Geometry: final body of the model. Coordinates: model frame, mm. Face numbers are marked on the shaded views. A direction names the side the tool comes from. Give positions to 0.01 mm unless a question says otherwise; leave off trailing zeros. Loops run counter-clockwise (first coordinate to the right, second up) from the corner with the lowest first, then second, coordinate; pieces in that order, holes last.
1. Section B-B, the plane y = 0. Output: boundary loops of the cut face in (x, z).
2. Access query for the marked faces 5, 6 and 7. Directions: +Z, -Z, +X, -X, +Y, -Y. A direction counts if a zero-diameter tool reaches every point of the face in a straight line with its end or side. Return the directions, or none.
3. Material intervals for line 1 along Z through (x, y) = (-16, -11); line 2 along Z through (x, y) = (-53, 55); line 3 along X through (y, z) = (60, -5.5), sorted ascending.
4. Draft query along Z for the marked faces 1, 2, 3 and 4. Return one class per face: +Z half, -Z half, draft (parallel to the pull), parting line (faces both ways), or undercut.
5. Section A-A, the plane x = -10. Output: boundary loops of the cut face in (y, z), then the cut area to 3 significant figures.
6. Section D-D, the plane x = -62.5. Output: boundary loops of the cut face in (y, z).
7. Section C-C, the plane z = -20. Output: boundary loops of the cut face in (x, y), then the cut area to 3 significant figures.
8. First-contact query: P1, Ø22, axis at x = -27.5, y = 18, coming from the +Z side; P2, Ø6, axis at x = -55.5, y = 23, coming from the +Z side; P3, Ø1, axis at x = -36.5, y = 46.5, coming from the -Z side; P4, Ø1, axis at y = 38.5, z = -32.5, coming from the +X side. Flat tips, straight axial feed; report the tip coordinate or a pass-through.
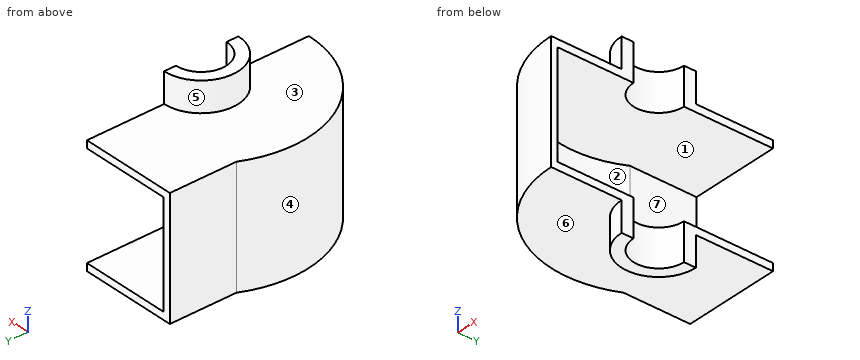
from build123d import *

# Parameters (mm, degrees)
BOSS_EXTRUDE1_DEPTH      = 20
BOSS_EXTRUDE1_DEPTH_BACK = 5
BOSS_EXTRUDE3_DEPTH      = 5
BOSS_EXTRUDE4_DEPTH      = 75


with BuildPart() as part:
    # Sketch1 → Boss-Extrude1 (new body, two sides)
    with BuildSketch(Plane.XY) as boss_extrude1_sk:
        with BuildLine():
            Line((0, 25), (0, 17))
            ThreePointArc((0, 17), (-17, 0), (0, -17))
            Line((0, -17), (0, -25))
            ThreePointArc((0, -25), (-25, 0), (0, 25))
        make_face()
    extrude(amount=BOSS_EXTRUDE1_DEPTH)
    extrude(boss_extrude1_sk.sketch, amount=-BOSS_EXTRUDE1_DEPTH_BACK)

    # Sketch2 → Boss-Extrude3 (add)
    with BuildSketch(Plane.XY):
        with BuildLine():
            Line((0, 25), (0, 77))
            Line((0, 77), (-65, 77))
            Line((-65, 77), (-65, 32.113081447))
            ThreePointArc((-65, 32.113081447), (-61.581037686, -38.262590053), (0, -72.5))
            Line((0, -72.5), (0, -25))
            ThreePointArc((0, -25), (-25, 0), (0, 25))
        make_face()
    extrude(amount=-BOSS_EXTRUDE3_DEPTH)


with BuildPart() as body_2:
    # Mirror7: mirrored copy
    add(part.part.mirror(Plane.XY.offset(-40)))


with BuildPart() as part_1:
    add(part.part)

    add(body_2.part)  # Boss-Extrude4 merges body 2
    # Sketch3 → Boss-Extrude4 (add)
    with BuildSketch(Plane.XY):
        with BuildLine():
            Line((-65, 32.113081447), (-65, 77))
            Line((-65, 77), (-60, 77))
            Line((-60, 77), (-60, 32.113081447))
            ThreePointArc((-60, 32.113081447), (-58.380864924, -34.970339014), (0, -68.053287944))
            Line((0, -68.053287944), (0, -72.5))
            ThreePointArc((0, -72.5), (-61.581037686, -38.262590053), (-65, 32.113081447))
        make_face()
    extrude(amount=-BOSS_EXTRUDE4_DEPTH)


solid = part_1.part
Answers below:
1. outline: (-72.5, -80) - (-25, -80) - (-25, -100) - (-17, -100) - (-17, -75) - (-68.05, -75) - (-68.05, -5) - (-17, -5) - (-17, 20) - (-25, 20) - (-25, 0) - (-72.5, 0) - close
2. face 5: +Z, -X
2. face 6: -Z, -X
2. face 7: +X, +Y
3. line 1: z = -100 to -75, -5 to 20
3. line 2: z = -80 to -75, -5 to 0
3. line 3: x = -65 to -60
4. face 1: undercut
4. face 2: undercut
4. face 3: +Z half
4. face 4: draft
5. outline: (-71.81, -80) - (-22.91, -80) - (-22.91, -100) - (-13.75, -100) - (-13.75, -75) - (-67.31, -75) - (-67.31, -5) - (-13.75, -5) - (-13.75, 20) - (-22.91, 20) - (-22.91, 0) - (-71.81, 0) - close; (13.75, -100) - (22.91, -100) - (22.91, -80) - (77, -80) - (77, -75) - (13.75, -75) - close; (13.75, -5) - (77, -5) - (77, 0) - (22.91, 0) - (22.91, 20) - (13.75, 20) - close
5. area: 2,260 mm2
6. outline: (-36.74, -80) - (77, -80) - (77, 0) - (-36.74, 0) - close; hole (-26.93, -75) - (26.93, -75) - (26.93, -5) - (-26.93, -5) - close
7. outline: (-65, 32.11) arc R72.5 ccw to (0, -72.5) - (0, -68.05) arc R68.05 cw to (-60, 32.11) - (-60, 77) - (-65, 77) - close
7. area: 864 mm2
8. P1: stops at z = 20
8. P2: stops at z = 0
8. P3: stops at z = -80
8. P4: stops at x = -60
